from build123d import *

# Parameters (mm, degrees)
SKETCH1_W           = 70
SKETCH1_H           = 19.05
BOSS_EXTRUDE1_DEPTH = 4
SKETCH2_W           = 70
SKETCH2_H           = 6.398717948
BOSS_EXTRUDE2_DEPTH = 15
FILLET1_R           = 2.54


with BuildPart() as part:
    # Sketch1 → Boss-Extrude1 (new body)
    with BuildSketch(Plane.XY):
        Rectangle(SKETCH1_W, SKETCH1_H)
    extrude(amount=BOSS_EXTRUDE1_DEPTH)

    # Sketch2 → Boss-Extrude2 (add)
    with BuildSketch(Plane.XY.offset(4)):
        Rectangle(SKETCH2_W, SKETCH2_H)
    extrude(amount=BOSS_EXTRUDE2_DEPTH)

    # Fillet1
    fillet1_edges = [part.edges().sort_by_distance(p)[0] for p in [
        (0, 3.199358974, 4),
        (0, -3.199358974, 4),
        (35, 0, 19),
        (0, 3.199358974, 19),
        (-35, 0, 19),
        (0, -3.199358974, 19),
        (35, -9.525, 2),
        (-35, -9.525, 2),
        (-35, 9.525, 2),
        (35, 9.525, 2),
    ]]
    fillet(fillet1_edges, radius=FILLET1_R)


solid = part.part
Verification items for the finished model (mm, model axes). A direction names the side the tool comes from. Give positions to 0.01 mm unless a question says otherwise; leave off trailing zeros. Order: outer loops, then holes, each group sorted by start corner. A loop starts at its lowest first (then second) coordinate and runs counter-clockwise, first axis right, second up. Notation, with made-up numbers: (-39.5, 7.25) -> (-4.5, 7.25) arc R19 ccw to (-4.5, 40.25) -> close; hole circle Ø5 at (66, 66.5). An arc over 180 degrees is marked (long way). Answer as CSV lines item,"result".
Q1. Depth check by flat-ended pin: pin 1 (2 mm diameter, centred on x = 25, y = 2, fed in from -Z); pin 2 (2 mm diameter, centred on x = 4, y = 6.5, fed in from +Z); pin 3 (4 mm diameter, centred on x = -25.5, z = 7, fed in from -Y); pin 4 (3 mm diameter, centred on x = 14.5, z = 13, fed in from +Y). Enter the tip coordinate at first touch or a pass-through.
Solutions:
pin 1,"stops at z = 0"
pin 2,"stops at z = 4.01"
pin 3,"stops at y = -3.72"
pin 4,"stops at y = 3.2"
Q2. Sectioned sample at A-A on x = 31.5. Record the cut outline in (y, z) (3 decimals).
Solutions:
outline,"(-9.525, 0) -> (9.525, 0) -> (9.525, 4) -> (5.739, 4) arc R2.54 cw to (3.199, 6.54) -> (3.199, 16.46) arc R2.54 ccw to (0.659, 19) -> (-0.659, 19) arc R2.54 ccw to (-3.199, 16.46) -> (-3.199, 6.54) arc R2.54 cw to (-5.739, 4) -> (-9.525, 4) -> close"
Q3. Release check for a two-part mould opening along Y. For faces 1 (the flat face through (0, 3.199, 11)), 2 (the cylindrical face through (0.49, -2.475, 18.236)), 3 (the flat face through (0, 8, 4)) record: +Y half, -Y half, draft (parallel to the pull), parting line (faces both ways), or undercut.
Solutions:
face 1,"+Y half"
face 2,"-Y half"
face 3,"draft"
Q4. Access from +Z, -Z, +X, -X, +Y, -Y to the whole of each face (thin tool, end or side, straight path). Record for faces 4 (the cylindrical face through (-34.56, 0.04, 17.89)), 5 (the flat face through (0, -3.199, 11)).
Solutions:
face 4,"+Z, -X, +Y, -Y"
face 5,"+Z, +X, -X, -Y"
Q5. Scan lines: probe 1 along Y at (x, z) = (26, 8.5); probe 2 along Z at (x, y) = (7.5, -0.75); probe 3 along Z at (x, y) = (-29, 8.75). Record each from-to range of solid material in increasing order.
Solutions:
probe 1,"y = -3.2 to 3.2"
probe 2,"z = 0 to 19"
probe 3,"z = 0 to 4"
Q6. Sectioned sample at C-C on y = -2.5. Record the cut outline in (x, z).
Solutions:
outline,"(-35, 0) -> (35, 0) -> (35, 16.46) arc R2.54 ccw to (34.3, 18.21) -> (-34.3, 18.21) arc R2.54 ccw to (-35, 16.46) -> close"
Q7. Sectioned sample at B-B on z = 14.5. Record the cut outline in (x, y).
Solutions:
outline,"(-35, -3.2) -> (35, -3.2) -> (35, 3.2) -> (-35, 3.2) -> close"
Q8. Sectioned sample at D-D on z = 4.75. Record the cut outline in (x, y).
Solutions:
outline,"(-35, -3.94) -> (35, -3.94) -> (35, 3.94) -> (-35, 3.94) -> close"
